Can you work these out from the model? Positions are in its coordinate system, mm. A direction names the side the tool comes from. Coordinates: 2 decimals unless noted, no trailing zeros. Loops run counter-clockwise (first coordinate to the right, second up) from the corner with the lowest first, then second, coordinate; pieces in that order, holes last. Notation, with made-up numbers: M 28,-13 L 75,-13 A20 ccw 75,21 Z; hole C 36,-7.75 d9. An arc over 180 degrees is marked long. Answer as a JSON object with one key per item and string values. Group by question number.
Item 1: Suppose I cut it at D-D (x = 21.75). Write out the boundary of the cut face in (y, z).
Item 2: If I drill on line 1 (X direction, y = 2.5, z = -4); line 2 (Y direction, x = 25.5, z = -23); line 3 (Z direction, x = 4.5, y = 8.5), over which ranges is the centre line in solid material (lowest first)?
Item 3: Suppose I cut it at A-A (y = 5.75). Write out the boundary of the cut face in (x, z).
Item 4: Suppose I cut it at C-C (z = -14.5). Write out the boundary of the cut face in (x, y).
Item 5: Which directions (+Z, -Z, +X, -X, +Y, -Y) give clear straight access to the entire face, cutting with the end or side of a thin tool? Please do faces 1 (the flat face through (6, 7, -2)), 2 (the flat face through (28, 7, -5)), 3 (the cylindrical face through (24.785, 7.07, -4.699)).
Item 6: I'm going to push flat-ended pins straight in: pin 1 Ø2 at (x, z) = (7, -26.5) entering from -Y; pin 2 Ø8 at (x, z) = (12.5, -27) entering from +Y; pin 3 Ø1.3 at (x, y) = (28.5, 8) entering from -Z. Where does each tip first touch, or does it pass through?
Item 7: Suppose I cut it at B-B (x = 26.5). Write out the boundary of the cut face in (y, z).
Item 8: We'd pull the mould along X, two halves only. Please class faces 4 (the cylindrical face through (5.715, 7.07, -4.699)), 5 (the flat face through (2, 7, -5)), 6 (the flat face through (30, 1.5, -12.6)): +X half, -X half, draft (parallel to the pull), parting line (faces both ways), or undercut.
```python
from build123d import *

# Parameters (mm, degrees)
SKETCH2_W           = 30
SKETCH2_H           = 34.29
BOSS_EXTRUDE1_DEPTH = 2
SKETCH3_W           = 5.5
SKETCH3_H           = 5
SKETCH3_W_2         = 6
BOSS_EXTRUDE2_DEPTH = 10
FILLET2_R           = 2
FILLET3_R           = 1


with BuildPart() as part:
    # Sketch2 → Boss-Extrude1 (new body)
    with BuildSketch(Plane(origin=(0, 0, 0), x_dir=(1, 0, 0), z_dir=(0, 1, 0))):
        with Locations((15, 17.145)):
            Rectangle(SKETCH2_W, SKETCH2_H)
    extrude(amount=BOSS_EXTRUDE1_DEPTH)

    # Sketch3 → Boss-Extrude2 (add)
    with BuildSketch(Plane(origin=(0, 2, 0), x_dir=(1, 0, 0), z_dir=(0, 1, 0))):
        with Locations((27.25, 2.5)):
            Rectangle(SKETCH3_W, SKETCH3_H)
        with Locations((3, 2.5)):
            Rectangle(SKETCH3_W_2, SKETCH3_H)
    extrude(amount=BOSS_EXTRUDE2_DEPTH)

    # Fillet2
    fillet2_edges = [part.edges().sort_by_distance(p)[0] for p in [
        (0, 1, -34.29),
        (30, 1, -34.29),
        (30, 6, 0),
        (0, 6, 0),
    ]]
    fillet(fillet2_edges, radius=FILLET2_R)

    # Fillet3
    fillet3_edges = [part.edges().sort_by_distance(p)[0] for p in [
        (24.5, 7, -5),
        (6, 7, -5),
    ]]
    fillet(fillet3_edges, radius=FILLET3_R)


solid = part.part
```
From the geometry:
{
 "1": {"outline": "M 0,-34.29 L 2,-34.29 L 2,0 L 0,0 Z"},
 "2": {"line 1": "0 to 6, 24.5 to 30", "line 2": "0 to 2", "line 3": "-5 to 0"},
 "3": {"outline": "M 0,-5 L 5,-5 A1 ccw 6,-4 L 6,0 L 2,0 A2 ccw 0,-2 Z; M 24.5,-4 A1 ccw 25.5,-5 L 30,-5 L 30,-2 A2 ccw 28,0 L 24.5,0 Z"},
 "4": {"outline": "M 0,0 L 30,0 L 30,2 L 0,2 Z"},
 "5": {"face 1": "+Z, -Z, +Y", "face 2": "-Z, +X, -X, +Y", "face 3": "-Z, +Y"},
 "6": {"pin 1": "y = 0", "pin 2": "y = 2", "pin 3": "z = -5"},
 "7": {"outline": "M 0,-34.29 L 2,-34.29 L 2,-5 L 12,-5 L 12,0 L 0,0 Z"},
 "8": {"face 4": "undercut", "face 5": "draft", "face 6": "+X half"}
}
